```python
from build123d import *

# Parameters (mm, degrees)
SKETCH001_W  = 7.6
SKETCH001_H  = 7.6
PAD001_DEPTH = 1.2
POCKET_DEPTH = 5
FILLET_R     = 0.15


with BuildPart() as part:
    # Sketch001 → Pad001 (new body)
    with BuildSketch(Plane.XY):
        Rectangle(SKETCH001_W, SKETCH001_H)
    extrude(amount=PAD001_DEPTH)

    # Sketch002 → Pocket (cut)
    with BuildSketch(Plane.XY.offset(1.2)):
        Polygon((-4.51175, 4.275026), (-1.233854, 4.275026), (-4.51175, 0.99713), align=None)
        Polygon((3.320655, 4.59318), (3.320655, 3.330028), (4.467743, 3.330028), align=None)
        Polygon((4.51175, -0.99713), (1.233854, -4.275026), (4.51175, -4.275026), align=None)
    extrude(amount=-POCKET_DEPTH, mode=Mode.SUBTRACT)

    # Fillet
    fillet_edges = [part.edges().sort_by_distance(p)[0] for p in [
        (-3.8, 1.70888, 0.6),
        (-3.8, -3.8, 0.6),
        (1.70888, -3.8, 0.6),
        (3.8, -1.70888, 0.6),
        (3.8, 3.330028, 0.6),
        (3.320655, 3.330028, 0.6),
        (3.320655, 3.8, 0.6),
        (-1.70888, 3.8, 0.6),
    ]]
    fillet(fillet_edges, radius=FILLET_R)


solid = part.part
```
Source: CAD feature listing. Evaluate the final solid. Frame: model axes, mm. Round coordinates to 2 decimals unless told otherwise and drop trailing zeros. Loops run counter-clockwise (first coordinate to the right, second up) from the corner with the lowest first, then second, coordinate; pieces in that order, holes last. Notation, with made-up numbers: M -13,23 L 41,23 A29 ccw 41,48 Z; hole C 71.25,69.5 d6. An arc over 180 degrees is marked long. Use a Markdown table: item, result. Add a question column.
1. Cut plane B-B, the plane x = 2.5. Output: boundary loops of the cut face in (y, z), and give its area (3 significant figures).
2. Cut plane C-C, the plane y = 2. Output: boundary loops of the cut face in (x, z).
3. Cut plane A-A, the plane z = 0.4. Output: boundary loops of the cut face in (x, y).
4. Ray query, line 1 along Y through (x, z) = (-1.75, 0.15); line 2 along X through (y, z) = (1.75, 0.1); line 3 along Y through (x, z) = (3.25, 0.9). Return the intervals inside material, ascending. Write a range as [from, to].
Solution:
| question | item | result |
|---|---|---|
| 1 | outline | M -3.01,0 L 3.8,0 L 3.8,1.2 L -3.01,1.2 Z |
| 1 | area | 8.17 mm2 |
| 2 | outline | M -3.51,0 L 3.8,0 L 3.8,1.2 L -3.51,1.2 Z |
| 3 | outline | M -3.8,-3.65 A0.15 ccw -3.65,-3.8 L 1.65,-3.8 A0.15 ccw 1.75,-3.76 L 3.76,-1.75 A0.15 ccw 3.8,-1.65 L 3.8,3.18 A0.15 ccw 3.65,3.33 L 3.47,3.33 A0.15 cw 3.32,3.48 L 3.32,3.65 A0.15 ccw 3.17,3.8 L -1.65,3.8 A0.15 ccw -1.75,3.76 L -3.76,1.75 A0.15 ccw -3.8,1.65 Z |
| 4 | line 1 | y = [-3.8, 3.76] |
| 4 | line 2 | x = [-3.76, 3.8] |
| 4 | line 3 | y = [-2.26, 3.78] |
